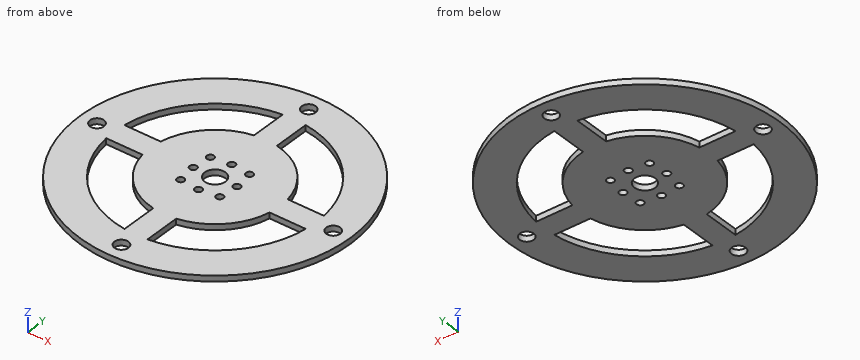
from build123d import *

# Parameters (mm, degrees)
SKETCH_2_R      = 47
SKETCH_2_R_2    = 2.425
SKETCH_2_R_3    = 35
SKETCH_2_R_4    = 22.5
SKETCH_2_R_5    = 1.25
SKETCH_2_R_6    = 3.6
EXTRUDE_1_DEPTH = 2


with BuildPart() as part:
    # 草图2 → 凸台-拉伸1 (new body)
    # profile 1 of 6: a face of its own
    with BuildSketch(Plane.XY):
        Circle(SKETCH_2_R)
        with Locations((-0.813609012, -41.166960847)):
            Circle(SKETCH_2_R_2, mode=Mode.SUBTRACT)
        Circle(SKETCH_2_R_3, mode=Mode.SUBTRACT)
        with Locations((0.813609012, 41.166960847)):
            Circle(SKETCH_2_R_2, mode=Mode.SUBTRACT)
        with Locations((41.166960847, -0.813609012)):
            Circle(SKETCH_2_R_2, mode=Mode.SUBTRACT)
        with Locations((-41.166960847, 0.813609012)):
            Circle(SKETCH_2_R_2, mode=Mode.SUBTRACT)
    # profile 2 of 6: a face of its own
    with BuildSketch(Plane.XY):
        with BuildLine():
            Line((-34.842927678, -3.312158032), (-22.21630595, -3.561706044))
            ThreePointArc((-22.21630595, -3.561706044), (-22.49560702, 0.444595088), (-22.058227696, 4.436732007))
            Line((-22.058227696, 4.436732007), (-34.684849424, 4.686280019))
            ThreePointArc((-34.684849424, 4.686280019), (-34.993166476, 0.69159236), (-34.842927678, -3.312158032))
        make_face()
    # profile 3 of 6: a face of its own
    with BuildSketch(Plane.XY):
        with BuildLine():
            Line((3.312158032, -34.842927678), (3.561706044, -22.21630595))
            ThreePointArc((3.561706044, -22.21630595), (-0.444595088, -22.49560702), (-4.436732007, -22.058227696))
            Line((-4.436732007, -22.058227696), (-4.686280019, -34.684849424))
            ThreePointArc((-4.686280019, -34.684849424), (-0.69159236, -34.993166476), (3.312158032, -34.842927678))
        make_face()
    # profile 4 of 6: a face of its own
    with BuildSketch(Plane.XY):
        with BuildLine():
            ThreePointArc((22.5, 0), (22.389284526, -2.229335869), (22.058227696, -4.436732007))
            Line((22.058227696, -4.436732007), (34.684849424, -4.686280019))
            ThreePointArc((34.684849424, -4.686280019), (34.921123477, -2.348432472), (35, 0))
            ThreePointArc((35, 0), (34.960709866, 1.657940179), (34.842927678, 3.312158032))
            Line((34.842927678, 3.312158032), (22.21630595, 3.561706044))
            ThreePointArc((22.21630595, 3.561706044), (22.428964353, 1.786493231), (22.5, 0))
        make_face()
    # profile 5 of 6: a face of its own
    with BuildSketch(Plane.XY):
        with BuildLine():
            Line((-3.312158032, 34.842927678), (-3.561706044, 22.21630595))
            ThreePointArc((-3.561706044, 22.21630595), (0.444595088, 22.49560702), (4.436732007, 22.058227696))
            Line((4.436732007, 22.058227696), (4.686280019, 34.684849424))
            ThreePointArc((4.686280019, 34.684849424), (0.69159236, 34.993166476), (-3.312158032, 34.842927678))
        make_face()
    # profile 6 of 6: a face of its own
    with BuildSketch(Plane.XY):
        Circle(SKETCH_2_R_4)
        with Locations((7.5, 0)):
            Circle(SKETCH_2_R_5, mode=Mode.SUBTRACT)
        with Locations((0, 7.5)):
            Circle(SKETCH_2_R_5, mode=Mode.SUBTRACT)
        with Locations((0, -7.5)):
            Circle(SKETCH_2_R_5, mode=Mode.SUBTRACT)
        with Locations((-6.717514421, 6.717514421)):
            Circle(SKETCH_2_R_5, mode=Mode.SUBTRACT)
        with Locations((-6.717514421, -6.717514421)):
            Circle(SKETCH_2_R_5, mode=Mode.SUBTRACT)
        with Locations((6.717514421, -6.717514421)):
            Circle(SKETCH_2_R_5, mode=Mode.SUBTRACT)
        with Locations((-7.5, 0)):
            Circle(SKETCH_2_R_5, mode=Mode.SUBTRACT)
        with Locations((6.717514421, 6.717514421)):
            Circle(SKETCH_2_R_5, mode=Mode.SUBTRACT)
        Circle(SKETCH_2_R_6, mode=Mode.SUBTRACT)
    extrude(amount=EXTRUDE_1_DEPTH)


solid = part.part
Can you work these out from the model? Positions are in its coordinate system, mm. Coordinates: 2 decimals unless noted, no trailing zeros. Write each loop counter-clockwise with the first axis right and the second up, starting at its lowest first coordinate (ties: lowest second). Pieces come first, ordered by that corner, then holes. Notation, with made-up numbers: (80.5, 33) -> (133.5, 33) arc R25 cw to (133.5, 68) -> close; hole circle Ø7 at (88.5, -3). An arc over 180 degrees is marked (long way). Write each question's results on one line, items separated by ' | '. Start each with the question number.
Item 1: I'm going to push a flat-ended pin straight in: P1, Ø1, axis at y = 9, z = 1.5, coming from the +X side (3 decimals). Where does the tip first touch, or does it pass through?
Item 2: If we section it at A-A, the plane y = -16: Write out the boundary of the cut face in (x, z), and give its area (3 significant figures).
Item 3: If we section it at B-B, the plane x = 18: Write out the boundary of the cut face in (y, z), and give its area (3 significant figures).
Item 4: If we section it at C-C, the plane z = 0.35: Count the separate pieces of the cut face and the enclosed holes in it, and give its area (3 significant figures).
Item 5: If we section it at D-D, the plane x = 0: Write out the boundary of the cut face in (y, z).
Item 6: Please list where these lines run through material, in increasing order: probe 1 along Y at (x, z) = (0, 0.95); probe 2 along X at (y, z) = (-2, 1.75); probe 3 along X at (y, z) = (31, 1.15).
Answer block:
1) P1: x = 46.225
2) outline: (-44.19, 0) -> (-31.13, 0) -> (-31.13, 2) -> (-44.19, 2) -> close; (-15.82, 0) -> (15.82, 0) -> (15.82, 2) -> (-15.82, 2) -> close; (31.13, 0) -> (44.19, 0) -> (44.19, 2) -> (31.13, 2) -> close | area: 116 mm²
3) outline: (-43.42, 0) -> (-30.02, 0) -> (-30.02, 2) -> (-43.42, 2) -> close; (-13.5, 0) -> (13.5, 0) -> (13.5, 2) -> (-13.5, 2) -> close; (30.02, 0) -> (43.42, 0) -> (43.42, 2) -> (30.02, 2) -> close | area: 108 mm²
4) separate pieces: 1 | enclosed holes: 17 | area: 4,930 mm²
5) outline: (-47, 0) -> (-43.45, 0) -> (-43.45, 2) -> (-47, 2) -> close; (-38.88, 0) -> (-8.75, 0) -> (-8.75, 2) -> (-38.88, 2) -> close; (-6.25, 0) -> (-3.6, 0) -> (-3.6, 2) -> (-6.25, 2) -> close; (3.6, 0) -> (6.25, 0) -> (6.25, 2) -> (3.6, 2) -> close; (8.75, 0) -> (38.88, 0) -> (38.88, 2) -> (8.75, 2) -> close; (43.45, 0) -> (47, 0) -> (47, 2) -> (43.45, 2) -> close
6) probe 1: -47 to -43.45, -38.88 to -8.75, -6.25 to -3.6, 3.6 to 6.25, 8.75 to 38.88, 43.45 to 47 | probe 2: -46.96 to -2.99, 2.99 to 39.05, 43.28 to 46.96 | probe 3: -35.33 to -16.25, -3.39 to 4.61, 16.25 to 35.33
